Design review of the part built by this model. Coordinates are the model's own, in mm. Face numbers are marked on the shaded views. Coordinates: 2 decimals unless noted, no trailing zeros. Write each loop counter-clockwise with the first axis right and the second up, starting at its lowest first coordinate (ties: lowest second). Pieces come first, ordered by that corner, then holes. Notation, with made-up numbers: M -35,20 L 4,20 A27 cw 4,55 Z; hole C -3.5,84.5 d6. An arc over 180 degrees is marked long. Write item = value, one per line.
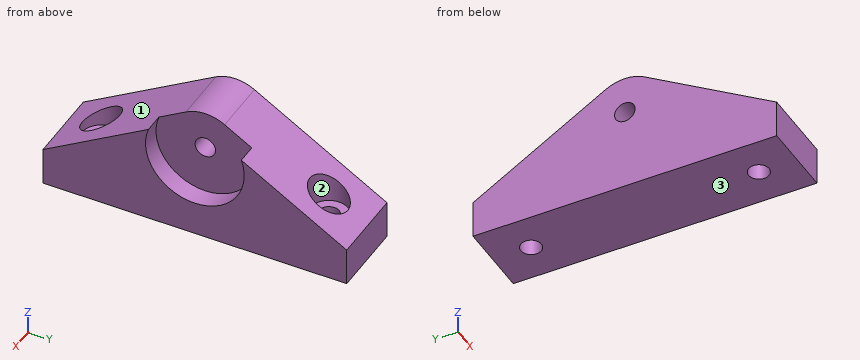
```python
from build123d import *

# Parameters (mm, degrees)
SKETCH1_W           = 20
SKETCH1_H           = 80
SKETCH1_R           = 2.7
BOSS_EXTRUDE1_DEPTH = 10
SKETCH2_R           = 2.7
BOSS_EXTRUDE2_DEPTH = 10
SKETCH3_R           = 5
CUT_EXTRUDE1_DEPTH  = 23
SKETCH4_R           = 13
CUT_EXTRUDE2_DEPTH  = 5.2


with BuildPart() as part:
    # Sketch1 → Boss-Extrude1 (new body)
    with BuildSketch(Plane.XY):
        with Locations((0, -30)):
            Rectangle(SKETCH1_W, SKETCH1_H)
        Circle(SKETCH1_R, mode=Mode.SUBTRACT)
        with Locations((0, -60)):
            Circle(SKETCH1_R, mode=Mode.SUBTRACT)
    extrude(amount=BOSS_EXTRUDE1_DEPTH)

    # Sketch2 → Boss-Extrude2 (add, symmetric)
    with BuildSketch(Plane(origin=(0, 0, 0), x_dir=(0, 0, -1), z_dir=(1, 0, 0))):
        with BuildLine():
            Line((-10, 10), (-30.611529786, -24.916541064))
            ThreePointArc((-30.611529786, -24.916541064), (-32, -30), (-30.611529786, -35.083458936))
            Line((-30.611529786, -35.083458936), (-10, -70))
            Line((-10, -70), (-10, 10))
        make_face()
        with Locations((-22, -30)):
            Circle(SKETCH2_R, mode=Mode.SUBTRACT)
    extrude(amount=BOSS_EXTRUDE2_DEPTH, both=True)

    # Sketch3 → Cut-Extrude1 (cut, through all)
    with BuildSketch(Plane(origin=(0, 0, 10), x_dir=(-1, 0, 0), z_dir=(0, 0, -1))):
        with Locations((0, -60)):
            Circle(SKETCH3_R)
        Circle(SKETCH3_R)
    extrude(amount=-CUT_EXTRUDE1_DEPTH, mode=Mode.SUBTRACT)

    # Sketch4 → Cut-Extrude2 (cut)
    with BuildSketch(Plane(origin=(10, 0, 0), x_dir=(0, 0, -1), z_dir=(1, 0, 0))):
        with Locations((-22, -30)):
            Circle(SKETCH4_R)
    extrude(amount=-CUT_EXTRUDE2_DEPTH, mode=Mode.SUBTRACT)


solid = part.part
```
Q1. Consider section A-A, the plane y = -30. State the section outline as (x, z) points.
Check result:
outline = M -10,0 L 10,0 L 10,9 L 4.8,9 L 4.8,19.3 L -10,19.3 Z; M -10,24.7 L 4.8,24.7 L 4.8,32 L -10,32 Z
Q2. Consider section D-D, the plane x = 8. State the section outline as (y, z) points.
Check result:
outline = M -70,0 L 10,0 L 10,10 L -17.76,26.39 A13 cw long -42.24,26.39 L -70,10 Z
Q3. The part is to be moulded in two halves that separate along Y. For the marked faces 1, 2 and 3, say which applies: +Y half, -Y half, draft (parallel to the pull), parting line (faces both ways), or undercut.
Check result:
face_1 = -Y half
face_2 = undercut
face_3 = draft
Q4. Wall thickness on line 1 (X direction, y = 0, z = 12.25); line 2 (Y direction, x = 0, z = 17.25); line 3 (Y direction, x = -5.75, z = 22): over which ranges is each line inside the solid? List them lowest first.
Check result:
line_1 = -10 to -5, 5 to 10
line_2 = -55 to -5
line_3 = -49.67 to -32.7, -27.3 to -10.33
Q5. Consider section C-C, the plane z = 12.5. State the section outline as (x, y) points.
Check result:
outline = M -10,-65.76 L 10,-65.76 L 10,-38.87 L 4.8,-38.87 L 4.8,-21.13 L 10,-21.13 L 10,5.76 L -10,5.76 Z; hole C 0,-60 d10; hole C 0,0 d10
Q6. For P1, Ø12, axis at x = 0, y = -60, coming from the -Z side; P2, Ø1, axis at x = 0, z = 23, coming from the +Y side; P3, Ø6, axis at x = 0.5, y = -10, coming from the +Z side; P4, Ø11.5, axis at x = 0, y = 0, coming from the +Z side, all flat-tipped, find the tip position at first contact; note any pin that passes through.
Check result:
P1 = 0
P2 = -11.18
P3 = 23.58
P4 = 19.3
Q7. Consider section B-B, the plane x = 1. State the section outline as (y, z) points (3 decimals).
Check result:
outline = M -70,0 L -62.508,0 L -62.508,10 L -64.899,10 L -64.899,13.011 L -70,10 Z; M -57.492,0 L -2.508,0 L -2.508,10 L -4.899,10 L -4.899,18.795 L -24.917,30.612 A10 ccw -35.083,30.612 L -55.101,18.795 L -55.101,10 L -57.492,10 Z; M 2.508,0 L 10,0 L 10,10 L 4.899,13.011 L 4.899,10 L 2.508,10 Z; hole C -30,22 d5.4
